The model under review builds one solid part; all positions refer to its coordinate system, in mm. Face numbers are marked on the shaded views. A direction names the side the tool comes from. Coordinates: 2 decimals unless noted, no trailing zeros. Loops run counter-clockwise (first coordinate to the right, second up) from the corner with the lowest first, then second, coordinate; pieces in that order, holes last. Notation, with made-up numbers: (-15.75, -25) - (36.25, -25) arc R22 cw to (36.25, -8) - close; hole circle Ø7 at (-14, -26). An arc over 180 degrees is marked (long way). Answer in a Markdown table with one row per item. Add a question column.
(1) We need section B-B on x = 59. Write out the cut boundary in (y, z).
(2) We need section A-A on y = 2.25. Write out the cut boundary in (x, z).
(3) We need section C-C on y = 17.25. Write out the cut boundary in (x, z) (3 decimals).
(4) We need section D-D on z = -64.5. Write out the cut boundary in (x, y).
(5) Machinability: for the marked faces 4, 5, 6 and 7, which of the approach directions +Z, -Z, +X, -X, +Y, -Y give a long, thin tool a straight path to every point of the face, cutting with its end or side? Answer none if there is none.
(6) For line 1 along X through (y, z) = (17.75, -77.5); line 2 along Z through (x, y) = (97.5, 14) (3 decimals); line 3 along Z through (x, y) = (51, 1), list the stretches that pass through material, from the lowest coordinate up.
(7) For P1, Ø6, axis at y = 16.5, z = -12.5, coming from the -X side; P2, Ø2, axis at x = 40.61, z = -77.5, coming from the +Y side; P3, Ø10, axis at x = 23, y = 9.5, coming from the -Z side; P4, Ø6, axis at y = 12, z = -66.5, coming from the +X side, all flat-tipped, find the tip position at first contact; note any pin that passes through.
(8) Mouldability with a two-part tool opening along X and no side actions: class the marked faces 1, 2 and 3 as +X half, -X half, draft (parallel to the pull), parting line (faces both ways), or undercut.
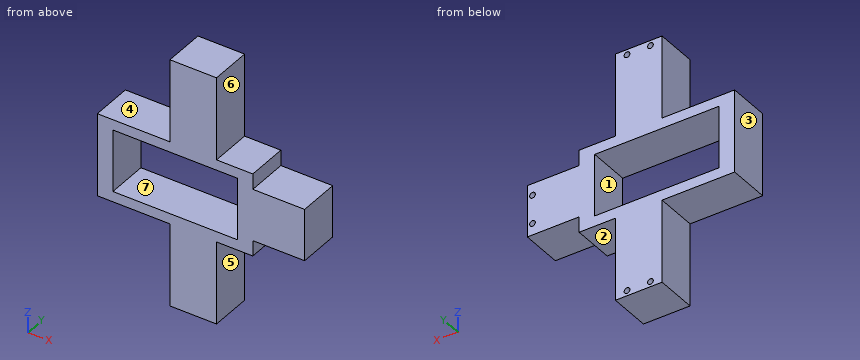
from build123d import *

# Parameters (mm, degrees)
BOSS_EXTRUDE1_DEPTH       = 20
CUT_EXTRUDE1_REACH        = 131.615
SKETCH3_W                 = 60
SKETCH3_H                 = 30
F_1_0MM_DOWEL_HOLE4_D     = 2.75
F_1_0MM_DOWEL_HOLE4_DEPTH = 10
F_1_0MM_DOWEL_HOLE4_TIP   = 0.826183351


with BuildPart() as part:
    # Sketch2 → Boss-Extrude1 (new body)
    with BuildSketch(Plane(origin=(0, 0, 0), x_dir=(1, 0, 0), z_dir=(0, 1, 0))):
        Polygon((57.5, 0), (57.5, -40), (35.013042541, -40), (35.013042541, 0), (0, 0), (0, 40), (35.013042541, 40), (35.013042541, 80), (57.5, 80), (57.5, 40), (75, 40), (75, 32.5), (100, 32.5), (100, 7.5), (75, 7.5), (75, 0), align=None)
    extrude(amount=BOSS_EXTRUDE1_DEPTH)

    # Sketch3 → Cut-Extrude1 (cut, up to next)
    with BuildSketch(Plane(origin=(0, 20, 0), x_dir=(1, 0, 0), z_dir=(0, 1, 0)), mode=Mode.PRIVATE) as cut_extrude1_sk1:
        with Locations((37.5, 20)):
            Rectangle(SKETCH3_W, SKETCH3_H)
    cut_extrude1_tool1 = extrude(cut_extrude1_sk1.sketch, amount=-CUT_EXTRUDE1_REACH, mode=Mode.PRIVATE) & part.part
    add(cut_extrude1_tool1.solids().sort_by_distance((37.5, 20, -20))[0], mode=Mode.SUBTRACT)

    # Ø1.0mm Dowel Hole4
    with Locations(Plane(origin=(0, 20, 0), x_dir=(1, 0, 0), z_dir=(0, 1, 0))):
        with Locations((51.90652127, 77.5), (40.60652127, -37.5), (51.90652127, -37.5), (97.5, 13.15), (97.5, 26.85), (40.60652127, 77.5)):
            Hole(F_1_0MM_DOWEL_HOLE4_D / 2, depth=F_1_0MM_DOWEL_HOLE4_DEPTH)
            with Locations((0, 0, -(F_1_0MM_DOWEL_HOLE4_DEPTH + F_1_0MM_DOWEL_HOLE4_TIP / 2))):  # 118° drill point
                Cone(0, F_1_0MM_DOWEL_HOLE4_D / 2, F_1_0MM_DOWEL_HOLE4_TIP, mode=Mode.SUBTRACT)


solid = part.part
Outcome:
| question | item | result |
|---|---|---|
| 1 | outline | (0, -40) - (20, -40) - (20, -35) - (0, -35) - close; (0, -5) - (20, -5) - (20, 0) - (0, 0) - close |
| 2 | outline | (0, -40) - (35.01, -40) - (35.01, -80) - (57.5, -80) - (57.5, -40) - (75, -40) - (75, -32.5) - (100, -32.5) - (100, -7.5) - (75, -7.5) - (75, 0) - (57.5, 0) - (57.5, 40) - (35.01, 40) - (35.01, 0) - (0, 0) - close; hole (7.5, -35) - (67.5, -35) - (67.5, -5) - (7.5, -5) - close |
| 3 | outline | (0, -40) - (35.013, -40) - (35.013, -80) - (57.5, -80) - (57.5, -40) - (75, -40) - (75, -32.5) - (100, -32.5) - (100, -7.5) - (75, -7.5) - (75, 0) - (57.5, 0) - (57.5, 40) - (35.013, 40) - (35.013, 0) - (0, 0) - close; hole (7.5, -35) - (67.5, -35) - (67.5, -5) - (7.5, -5) - close; hole circle Ø2.75 at (40.607, -77.5); hole circle Ø2.75 at (40.607, 37.5); hole circle Ø2.75 at (51.907, -77.5); hole circle Ø2.75 at (51.907, 37.5); hole circle Ø2.75 at (97.5, -26.85); hole circle Ø2.75 at (97.5, -13.15) |
| 4 | outline | (35.01, 0) - (57.5, 0) - (57.5, 20) - (35.01, 20) - close |
| 5 | face 4 | +Z, -X, +Y, -Y |
| 5 | face 5 | -Z, +X, +Y, -Y |
| 5 | face 6 | +Z, +X, +Y, -Y |
| 5 | face 7 | +Y, -Y |
| 6 | line 1 | 35.01 to 39.23, 41.98 to 50.53, 53.28 to 57.5 |
| 6 | line 2 | -32.5 to -28.225, -25.475 to -14.525, -11.775 to -7.5 |
| 6 | line 3 | -80 to -35, -5 to 40 |
| 7 | P1 | x = 0 |
| 7 | P2 | y = 9.78 |
| 7 | P3 | z = -40 |
| 7 | P4 | x = 57.5 |
| 8 | face 1 | undercut |
| 8 | face 2 | draft |
| 8 | face 3 | -X half |
